from build123d import *

# Parameters (mm, degrees)
F0_W     = 1815
F0_H     = 1025
F0_W_2   = 545
F0_H_2   = 597.5
F0_H_3   = 935
F0_H_4   = 292.5
F1_DEPTH = 50
F2_W     = 15
F2_H     = 292.5
F3_DEPTH = 20


with BuildPart() as f1:
    # F0 (on Front) → F1 (new body)
    with BuildSketch(Plane.XZ):
        with Locations((907.5, 512.5)):
            Rectangle(F0_W, F0_H)
        with Locations((907.5, 343.75)):
            Rectangle(F0_W_2, F0_H_2, mode=Mode.SUBTRACT)
        with Locations((317.5, 512.5)):
            Rectangle(F0_W_2, F0_H_3, mode=Mode.SUBTRACT)
        with Locations((907.5, 833.75)):
            Rectangle(F0_W_2, F0_H_4, mode=Mode.SUBTRACT)
        with Locations((1497.5, 512.5)):
            Rectangle(F0_W_2, F0_H_3, mode=Mode.SUBTRACT)
    extrude(amount=F1_DEPTH)

    # F2 (on Front) → F3 (join)
    with BuildSketch(Plane.XZ):
        Polygon((325, 980), (310, 980), (310, 678.333333), (45, 678.333333), (45, 663.333333), (310, 663.333333), (310, 361.666667), (45, 361.666667), (45, 346.666667), (310, 346.666667), (310, 45), (327.010195, 45), (326.36163, 346.666667), (590, 346.666667), (590, 361.666667), (326.329381, 361.666667), (325.680815, 663.333333), (590, 663.333333), (590, 678.333333), (325.648566, 678.333333), align=None)
        Polygon((1498.095772, 980), (1483.095772, 980), (1483.095772, 678.333333), (1225, 678.333333), (1225, 663.333333), (1483.095772, 663.333333), (1483.095772, 361.666667), (1225, 361.666667), (1225, 346.666667), (1483.095772, 346.666667), (1483.095772, 45), (1498.095772, 45), (1498.095772, 346.666667), (1770, 346.666667), (1770, 361.666667), (1498.095772, 361.666667), (1498.095772, 663.333333), (1770, 663.333333), (1770, 678.333333), (1498.095772, 678.333333), align=None)
        with Locations((907.5, 833.75)):
            Rectangle(F2_W, F2_H)
        Polygon((915, 642.5), (900, 642.5), (900, 361.666667), (635, 361.666667), (635, 346.666667), (900, 346.666667), (900, 45), (915, 45), (915, 346.666667), (1180, 346.666667), (1180, 361.666667), (915, 361.666667), align=None)
    extrude(amount=F3_DEPTH)


solid = f1.part
Input: part model. Units: mm. Frame: model coordinates. A direction names the side the tool comes from. Coordinates: 2 decimals unless noted, no trailing zeros. Loops run counter-clockwise (first coordinate to the right, second up) from the corner with the lowest first, then second, coordinate; pieces in that order, holes last.
(1) Set-up query: faces 1 (the face through (635, -25, 832)), 2 (the face through (316, -20, 515)), 3 (the face through (0, -25, 505)). Return all of +Z, -Z, +X, -X, +Y, -Y with unobstructed straight access to the full face (end or side cutting, diameter ignored); none if empty.
(2) Section A-A on x = 470.5. Return the cut outline in (y, z).
(3) Material intervals for probe 1 along Z at (x, y) = (1000.5, -39); probe 2 along X at (y, z) = (-38, 705.5); probe 3 along Z at (x, y) = (1431, -19), sorted ascending.
(4) Section B-B on y = -29.5. Return the cut outline in (x, z).
(5) Pull-direction query (Z, two-part tool) for faces 4 (the face through (903, 0, 515)), 5 (the face through (906, -20, 345)), 6 (the face through (895, -25, 0)); classes: released by +Z, released by -Z, zero draft, split by the parting line, or undercut.
(6) Section D-D on x = 773.5. Return the cut outline in (y, z).
(7) Section C-C on z = 281. Return the cut outline in (x, y), then the cut area to 3 significant figures.
Data:
1. face 1: +Y, -Y
1. face 2: -Y
1. face 3: +Z, -Z, -X, +Y, -Y
2. outline: (-50, 0) - (0, 0) - (0, 45) - (-50, 45) - close; (-50, 980) - (0, 980) - (0, 1025) - (-50, 1025) - close; (-20, 346.67) - (0, 346.67) - (0, 361.67) - (-20, 361.67) - close; (-20, 663.33) - (0, 663.33) - (0, 678.33) - (-20, 678.33) - close
3. probe 1: z = 0 to 45, 642.5 to 687.5, 980 to 1025
3. probe 2: x = 0 to 45, 590 to 635, 1180 to 1225, 1770 to 1815
3. probe 3: z = 0 to 45, 346.67 to 361.67, 663.33 to 678.33, 980 to 1025
4. outline: (0, 0) - (1815, 0) - (1815, 1025) - (0, 1025) - close; hole (45, 45) - (590, 45) - (590, 980) - (45, 980) - close; hole (635, 45) - (1180, 45) - (1180, 642.5) - (635, 642.5) - close; hole (635, 687.5) - (1180, 687.5) - (1180, 980) - (635, 980) - close; hole (1225, 45) - (1770, 45) - (1770, 980) - (1225, 980) - close
5. face 4: zero draft
5. face 5: undercut
5. face 6: released by -Z
6. outline: (-50, 0) - (0, 0) - (0, 45) - (-50, 45) - close; (-50, 642.5) - (0, 642.5) - (0, 687.5) - (-50, 687.5) - close; (-50, 980) - (0, 980) - (0, 1025) - (-50, 1025) - close; (-20, 346.67) - (0, 346.67) - (0, 361.67) - (-20, 361.67) - close
7. outline: (0, -50) - (45, -50) - (45, 0) - (0, 0) - close; (310, -20) - (326.5, -20) - (326.5, 0) - (310, 0) - close; (590, -50) - (635, -50) - (635, 0) - (590, 0) - close; (900, -20) - (915, -20) - (915, 0) - (900, 0) - close; (1180, -50) - (1225, -50) - (1225, 0) - (1180, 0) - close; (1483.1, -20) - (1498.1, -20) - (1498.1, 0) - (1483.1, 0) - close; (1770, -50) - (1815, -50) - (1815, 0) - (1770, 0) - close
7. area: 9,930 mm2
